```python
from build123d import *

# Parameters (mm, degrees)
F0_W     = 15.6047875062
F0_H     = 36.0328741372
F1_DEPTH = 7.62
F2_SIZE  = 7.61999
F3_R     = 4.2995581312
F4_DEPTH = 0.5588


# Not quite as in the source:
# - a fillet or chamfer is up to 0.001 mm smaller than in the source, because OpenCascade refuses the exact size


with BuildPart() as f1:
    # F0 (on Top) → F1 (new body)
    with BuildSketch(Plane.XY):
        Rectangle(F0_W, F0_H)
    extrude(amount=F1_DEPTH)

    # F2 (size 7.62 in the source; OpenCascade refuses exactly that, so slightly less here)
    f2_edges = [f1.edges().sort_by_distance(p)[0] for p in [
        (0, -18.016437, 0),
    ]]
    chamfer(f2_edges, length=F2_SIZE)

    # F3 (on face) → F4 (join)
    with BuildSketch(Plane.XY.offset(7.62)):
        Circle(F3_R)
    extrude(amount=F4_DEPTH)


solid = f1.part
```
Work out the finished part from the listing and answer in its coordinate system (mm). A direction names the side the tool comes from. Coordinates: 2 decimals unless noted, no trailing zeros. Write each loop counter-clockwise with the first axis right and the second up, starting at its lowest first coordinate (ties: lowest second). Pieces come first, ordered by that corner, then holes.
Q1. A cutting plane is placed at D-D, the plane y = 7.5. Give the vertices of the cut face in (x, z), then the cut area to 3 significant figures.
Q2. A cutting plane is placed at C-C, the plane z = 4. Give the vertices of the cut face in (x, y), then the cut area to 3 significant figures.
Q3. A cutting plane is placed at B-B, the plane y = 0. Give the vertices of the cut face in (x, z), then the cut area to 3 significant figures.
Q4. Find the intervals of material crossed by line 1 (Z direction, x = 0.25, y = 14); line 2 (Y direction, x = -1.75, z = 6.25); line 3 (Y direction, x = 1.75, z = 2.25), in increasing order.
Q5. Each of these flat-tipped pins is pushed along its axis until it touches: pin 1 Ø4 at (x, z) = (6, 5) entering from -Y; pin 2 Ø3 at (x, y) = (2.5, -12.5) entering from +Z. Where does it stop, or does it pass through?
Q6. Which of the six approach directions +Z, -Z, +X, -X, +Y, -Y give full straight-line access (tool end or side, diameter ignored) to faces 1 (the face through (0, 0, 8.179)), 2 (the face through (-0.932, -4.197, 7.895))?
Findings below:
1. outline: (-7.8, 0) - (7.8, 0) - (7.8, 7.62) - (-7.8, 7.62) - close
1. area: 119 mm2
2. outline: (-7.8, -14.4) - (7.8, -14.4) - (7.8, 18.02) - (-7.8, 18.02) - close
2. area: 506 mm2
3. outline: (-7.8, 0) - (7.8, 0) - (7.8, 7.62) - (4.3, 7.62) - (4.3, 8.18) - (-4.3, 8.18) - (-4.3, 7.62) - (-7.8, 7.62) - close
3. area: 124 mm2
4. line 1: z = 0 to 7.62
4. line 2: y = -16.65 to 18.02
4. line 3: y = -12.65 to 18.02
5. pin 1: stops at y = -17.4
5. pin 2: stops at z = 7.62
6. face 1: +Z, +X, -X, +Y, -Y
6. face 2: +Z
